Answer from the drawing. Dimensions are ordinates in mm from the lowest x, y and z of the part. A direction names the side the tool comes from. Round coordinates to 2 decimals unless told otherwise and drop trailing zeros. Write each loop counter-clockwise with the first axis right and the second up, starting at its lowest first coordinate (ties: lowest second). Pieces come first, ordered by that corner, then holes. Notation, with made-up numbers: (70.25, -24.75) - (84.25, -24.75) arc R15 cw to (84.25, -16.75) - close; hole circle Ø4 at (1.5, 77.5). An arc over 180 degrees is marked (long way). Answer in a Markdown table with one row per item.
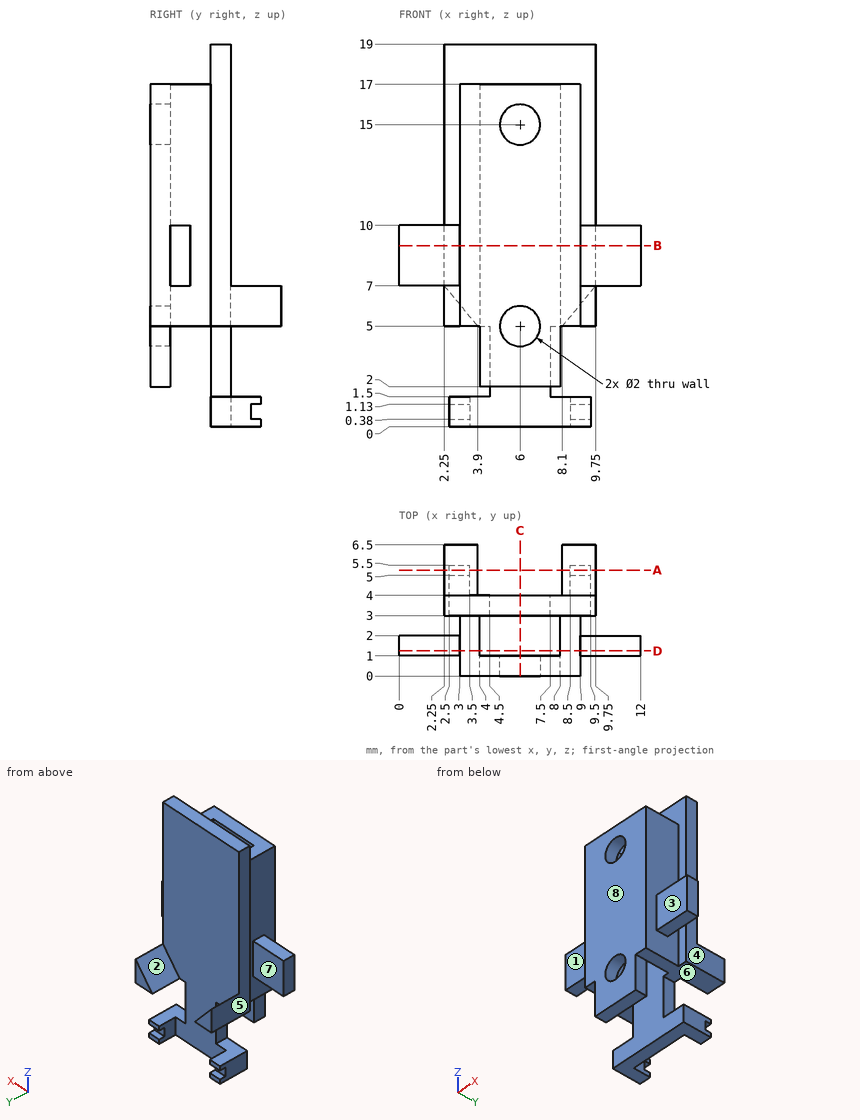
(1) Section B-B (z = 9) is taken. Give the vertices of the cut face in (x, y), and give its area (3 significant figures).
Checked values:
| item | result |
|---|---|
| outline | (0, 1) - (3, 1) - (3, 0) - (9, 0) - (9, 1) - (12, 1) - (12, 2) - (9, 2) - (9, 3) - (9.75, 3) - (9.75, 4) - (2.25, 4) - (2.25, 3) - (3, 3) - (3, 2) - (0, 2) - close; hole (4, 1) - (8, 1) - (8, 3) - (4, 3) - close |
| area | 23.5 mm2 |
(2) Find the intervals of material crossed by line 1 (Z direction, x = 6, y = 0.5); line 2 (Z direction, x = 8.25, y = 3.25); line 3 (X direction, y = 2, z = 11.5), in increasing order.
Checked values:
| item | result |
|---|---|
| line 1 | z = 2 to 4, 6 to 14, 16 to 17 |
| line 2 | z = 0 to 1.5, 5 to 19 |
| line 3 | x = 3 to 4, 8 to 9 |
(3) For a pull along Y with two mould halves and no side action, classify the marked faces 6, 7 and 8 as pulls with the +Y half, pulls with the -Y half, needs draft (parallel to the pull), parting line crosses it, or undercut.
Checked values:
| item | result |
|---|---|
| face 6 | needs draft |
| face 7 | undercut |
| face 8 | pulls with the -Y half |
(4) Flat-ended cylindrical pins translate along their axes: pin 1 (0.5 mm diameter, centred on y = 0.5, z = 4, fed in from +X); pin 2 (2 mm diameter, centred on x = 8.5, y = 4.5, fed in from +Z); pin 3 (0.8 mm diameter, centred on y = 5, z = 0.5, fed in from +X); pin 4 (4 mm diameter, centred on x = 10, z = 12, fed in from +Y). Find the tip coordinate at first contact, or state that the pin passes through.
Checked values:
| item | result |
|---|---|
| pin 1 | stops at x = 8 |
| pin 2 | stops at z = 19 |
| pin 3 | stops at x = 9.5 |
| pin 4 | stops at y = 4 |
(5) For the marked faces 1, 2, 3, 4 and 5, determine the directions among +Z, -Z, +X, -X, +Y, -Y from which every point of the face is accessible in a straight line to the end or side of a thin tool.
Checked values:
| item | result |
|---|---|
| face 1 | +Z, -Z, -X, -Y |
| face 2 | +Z, +Y |
| face 3 | +Z, -Z, +X, -Y |
| face 4 | +Z, -Z, +X, +Y |
| face 5 | +Z, -Z, -X, +Y |
(6) Section D-D (y = 1.25) is taken. Give the vertices of the cut face in (x, z).
Checked values:
| item | result |
|---|---|
| outline | (0, 7) - (3, 7) - (3, 5) - (4, 5) - (4, 17) - (3, 17) - (3, 10) - (0, 10) - close; (8, 5) - (9, 5) - (9, 7) - (12, 7) - (12, 10) - (9, 10) - (9, 17) - (8, 17) - close |
(7) Section C-C (x = 6) is taken. Give the vertices of the cut face in (y, z).
Checked values:
| item | result |
|---|---|
| outline | (0, 2) - (1, 2) - (1, 4) - (0, 4) - close; (0, 6) - (1, 6) - (1, 14) - (0, 14) - close; (0, 16) - (1, 16) - (1, 17) - (0, 17) - close; (3, 0) - (4, 0) - (4, 19) - (3, 19) - close |
(8) Section A-A (y = 5.25) is taken. Give the vertices of the cut face in (x, z).
Checked values:
| item | result |
|---|---|
| outline | (2.25, 5) - (3.9, 5) - (2.25, 7) - close; (2.5, 0) - (3.5, 0) - (3.5, 0.38) - (2.5, 0.38) - close; (2.5, 1.13) - (3.5, 1.13) - (3.5, 1.5) - (2.5, 1.5) - close; (8.1, 5) - (9.75, 5) - (9.75, 7) - close; (8.5, 0) - (9.5, 0) - (9.5, 0.38) - (8.5, 0.38) - close; (8.5, 1.13) - (9.5, 1.13) - (9.5, 1.5) - (8.5, 1.5) - close |
